Geometry check sheet. Reference: the model listing, model coordinates, mm. Face numbers are marked on the shaded views. A direction names the side the tool comes from. Give positions to 0.01 mm unless a question says otherwise; leave off trailing zeros. Order: outer loops, then holes, each group sorted by start corner. A loop starts at its lowest first (then second) coordinate and runs counter-clockwise, first axis right, second up. Notation, with made-up numbers: (-36.75, 30.25) - (-14.75, 30.25) arc R25 ccw to (-14.75, 58.25) - close; hole circle Ø2 at (27, -5). An arc over 180 degrees is marked (long way). Put each result on its own line as item: value. Start each with the question number.
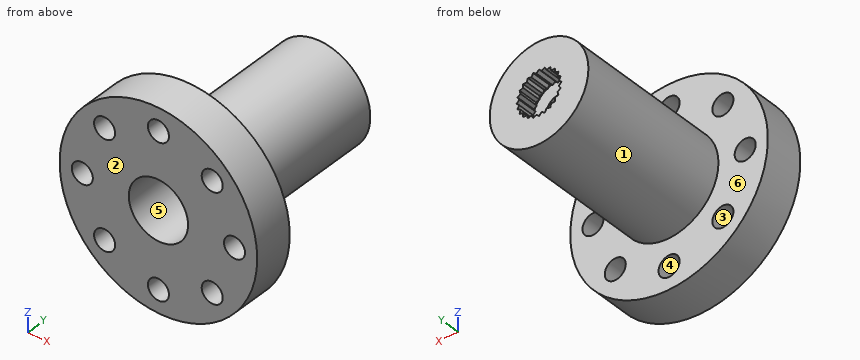
```python
from build123d import *

# Parameters (mm, degrees)
SKETCH1_W                  = 12.69619
SKETCH1_H                  = 5.08
SKETCH2_R                  = 6.34619
BOSS_EXTRUDE1_DEPTH        = 20.32
SKETCH3_R                  = 3.26136
CUT_EXTRUDE1_DEPTH         = 0.508
CUT_EXTRUDE2_REACH         = 27.4
SKETCH5_R                  = 3.81
CUT_EXTRUDE3_DEPTH         = 21.082
SKETCH6_R                  = 1.5
CUT_EXTRUDE4_DEPTH         = 5.318
M2_5_CLEARANCE_HOLE1_D     = 2.7051
M2_5_CLEARANCE_HOLE1_DEPTH = 5.08


with BuildPart() as part:
    # Sketch1 → Revolve1 (revolve)
    with BuildSketch(Plane.XY):
        with Locations((6.348095, 2.54)):
            Rectangle(SKETCH1_W, SKETCH1_H)
    revolve(axis=Axis((0, 5.08, 0), (0, -1, 0)))

    # Sketch2 → Boss-Extrude1 (add)
    with BuildSketch(Plane(origin=(0, 5.08, 0), x_dir=(-1, 0, 0), z_dir=(0, 1, 0))):
        Circle(SKETCH2_R)
    extrude(amount=BOSS_EXTRUDE1_DEPTH)

    # Sketch3 → Cut-Extrude1 (cut)
    with BuildSketch(Plane.XZ.offset(-22.352)):
        Circle(SKETCH3_R)
    extrude(amount=-CUT_EXTRUDE1_DEPTH, mode=Mode.SUBTRACT)

    # Sketch4 → Cut-Extrude2 (cut, up to next)
    with BuildSketch(Plane(origin=(0, 25.4, 0), x_dir=(-1, 0, 0), z_dir=(0, 1, 0)), mode=Mode.PRIVATE) as cut_extrude2_sk1:
        Polygon((-2.494464932, -1.44018), (-2.035268659, -1.56171657), (-2.036722088, -2.036722088), (-1.56171657, -2.035268659), (-1.44018, -2.494464932), (-0.981736077, -2.370120553), (-0.745492025, -2.782214113), (-0.334851894, -2.543452647), (0, -2.88036), (0.334851894, -2.543452647), (0.745492025, -2.782214113), (0.981736077, -2.370120553), (1.44018, -2.494464932), (1.56171657, -2.035268659), (2.036722088, -2.036722088), (2.035268659, -1.56171657), (2.494464932, -1.44018), (2.370120553, -0.981736077), (2.782214113, -0.745492025), (2.543452647, -0.334851894), (2.88036, 0), (2.543452647, 0.334851894), (2.782214113, 0.745492025), (2.370120553, 0.981736077), (2.494464932, 1.44018), (2.035268659, 1.56171657), (2.036722088, 2.036722088), (1.56171657, 2.035268659), (1.44018, 2.494464932), (0.981736077, 2.370120553), (0.745492025, 2.782214113), (0.334851894, 2.543452647), (0, 2.88036), (-0.334851894, 2.543452647), (-0.745492025, 2.782214113), (-0.981736077, 2.370120553), (-1.44018, 2.494464932), (-1.56171657, 2.035268659), (-2.036722088, 2.036722088), (-2.035268659, 1.56171657), (-2.494464932, 1.44018), (-2.370120553, 0.981736077), (-2.782214113, 0.745492025), (-2.543452647, 0.334851894), (-2.88036, 0), (-2.543452647, -0.334851894), (-2.782214113, -0.745492025), (-2.370120553, -0.981736077), align=None)
    cut_extrude2_tool1 = extrude(cut_extrude2_sk1.sketch, amount=-CUT_EXTRUDE2_REACH, mode=Mode.PRIVATE) & part.part
    add(cut_extrude2_tool1.solids().sort_by_distance((0, 25.4, 0))[0], mode=Mode.SUBTRACT)

    # Sketch5 → Cut-Extrude3 (cut)
    with BuildSketch(Plane.XZ):
        Circle(SKETCH5_R)
    extrude(amount=-CUT_EXTRUDE3_DEPTH, mode=Mode.SUBTRACT)

    # Sketch6 → Cut-Extrude4 (cut, through all)
    with BuildSketch(Plane.XZ.offset(-21.082)):
        Circle(SKETCH6_R)
    extrude(amount=-CUT_EXTRUDE4_DEPTH, mode=Mode.SUBTRACT)

    # M2.5 Clearance Hole1
    with Locations(Plane(origin=(0, 5.08, 0), x_dir=(1, 0, 0), z_dir=(0, 1, 0))):
        with Locations((6.914797213, -6.914797213), (0, -9.779), (-6.914797213, -6.914797213), (-9.779, 0), (-6.914797213, 6.914797213), (0, 9.779), (6.914797213, 6.914797213), (9.779, 0)):
            Hole(M2_5_CLEARANCE_HOLE1_D / 2, depth=M2_5_CLEARANCE_HOLE1_DEPTH)


solid = part.part
```
Item 1: Cross-section at B-B (y = 16). Enter the section's corners in (x, z), and give its area (3 significant figures).
Item 2: Cross-section at A-A (y = 2.25). Count the separate pieces of the cut face and the enclosed holes in it, and give its area (3 significant figures).
Item 3: Set-up check for the marked faces 4, 5 and 6: record each of +Z, -Z, +X, -X, +Y, -Y from which the full face is reachable in a straight line by a thin tool's end or side.
Item 4: Release check for a two-part mould opening along X. For the marked faces 1, 2 and 3 record: +X half, -X half, draft (parallel to the pull), parting line (faces both ways), or undercut.
Item 5: Gauge pin test, flat ends, axial feed: pin 1 Ø8.5 at (x, z) = (0, 0) entering from +Y; pin 2 Ø4 at (x, z) = (-1, 0) entering from -Y; pin 3 Ø12 at (x, y) = (4, 17.5) entering from -Z; pin 4 Ø1 at (y, z) = (5.5, 1.5) entering from +X. Record the tip position at first contact, or that the pin passes through.
Item 6: Thickness scan on line 1 along Z through (x, y) = (0, 2.15); line 2 along Z through (x, y) = (0, 22.7); line 3 along Z through (x, y) = (0.25, 8.5). Record the ranges inside material, lowest first.
Recorded:
1. outline: circle Ø12.69 at (0, 0); hole circle Ø7.62 at (0, 0)
1. area: 80.9 mm^2
2. separate pieces: 1
2. enclosed holes: 9
2. area: 415 mm^2
3. face 4: +Y, -Y
3. face 5: -Y
3. face 6: +Y
4. face 1: parting line
4. face 2: draft
4. face 3: undercut
5. pin 1: stops at y = 25.4
5. pin 2: stops at y = 21.08
5. pin 3: stops at z = -6.35
5. pin 4: stops at x = 12.64
6. line 1: z = -12.7 to -11.13, -8.43 to -3.81, 3.81 to 8.43, 11.13 to 12.7
6. line 2: z = -6.35 to -3.26, 3.26 to 6.35
6. line 3: z = -6.34 to -3.8, 3.8 to 6.34
